Part model, mm, in its own coordinate system. A direction names the side the tool comes from. Round coordinates to 2 decimals unless told otherwise and drop trailing zeros. Write each loop counter-clockwise with the first axis right and the second up, starting at its lowest first coordinate (ties: lowest second). Pieces come first, ordered by that corner, then holes. Notation, with made-up numbers: (10.25, 63) -> (59.25, 63) arc R20 cw to (59.25, 92) -> close; hole circle Ø8 at (51.5, 48.25). An arc over 180 degrees is marked (long way). Return JSON: item names as keys, results as strings. Group by question number.
(1) Tool access for faces 4 (the flat face through (0, -8, 0)), 5 (the flat face through (-2, -18, 2)), 6 (the flat face through (5, -17, 0)): list every direction of +Z, -Z, +X, -X, +Y, -Y with a clear straight run to the whole face (end or side of a thin tool).
(2) Mould opens along X. For faces 1 (the flat face through (-0.1, -17.3, -5)), 2 (the cylindrical face through (-2.44, -13.07, 0.54)), 3 (the flat face through (-5, -17, 0)) say: +X half, -X half, draft (parallel to the pull), parting line (faces both ways), or undercut.
(3) Drill centre lines: L1, parallel to Y at x = 0.5, z = 37.5; L2, parallel to X at y = -13, z = 0; L3, parallel to X at y = -10.25, z = 0. Where is each one in solid material? Low to high. Write a range as from..to.
(4) Saw through at B-B (x = 0). List the corners of the cut face in (y, z).
(5) Saw through at C-C (z = 0). List the corners of the cut face in (x, y), plus the area to 3 significant figures.
(6) Saw through at A-A (y = -15). List the corners of the cut face in (x, z).
(7) Drop flat-ended pins along their axis: pin 1 Ø2 at (x, z) = (-5, -26) entering from -Y; pin 2 Ø2 at (x, z) = (8.5, -25) entering from +Y; pin 3 Ø1.5 at (x, z) = (0, 0.5) entering from -Y. Give the stop position or say it passes through.
(8) Saw through at D-D (y = 14). List the corners of the cut face in (x, z).
from build123d import *

# Parameters (mm, degrees)
SKETCH1_R           = 17
BOSS_EXTRUDE1_DEPTH = 40
SKETCH2_W           = 10
SKETCH2_H           = 2
BOSS_EXTRUDE2_DEPTH = 5
SKETCH3_R           = 2.5
CUT_EXTRUDE1_DEPTH  = 10


with BuildPart() as part:
    # Sketch1 → Boss-Extrude1 (new, symmetric)
    with BuildSketch(Plane.XY):
        Circle(SKETCH1_R)
    extrude(amount=BOSS_EXTRUDE1_DEPTH, both=True)

    # Sketch2 → Boss-Extrude2 (add, symmetric)
    with BuildSketch(Plane.XY):
        with Locations((0, -17)):
            Rectangle(SKETCH2_W, SKETCH2_H)
    extrude(amount=BOSS_EXTRUDE2_DEPTH, both=True)

    # Sketch3 → Cut-Extrude1 (cut)
    with BuildSketch(Plane.XZ.offset(18)):
        with Locations(Location((0, 0, 0), (0, 0, 270))):
            Circle(SKETCH3_R)
    extrude(amount=-CUT_EXTRUDE1_DEPTH, mode=Mode.SUBTRACT)


solid = part.part
Computed values:
{
 "1": {"face 4": "-Y", "face 5": "+Z, -Z, +X, -X, -Y", "face 6": "+Z, -Z, +X, -Y"},
 "2": {"face 1": "draft", "face 2": "undercut", "face 3": "-X half"},
 "3": {"L1": "-16.99..16.99", "L2": "-10.95..-2.5, 2.5..10.95", "L3": "-13.56..-2.5, 2.5..13.56"},
 "4": {"outline": "(-18, -5) -> (-17, -5) -> (-17, -40) -> (17, -40) -> (17, 40) -> (-17, 40) -> (-17, 5) -> (-18, 5) -> (-18, 2.5) -> (-8, 2.5) -> (-8, -2.5) -> (-18, -2.5) -> close"},
 "5": {"outline": "(-5, -18) -> (-2.5, -18) -> (-2.5, -8) -> (2.5, -8) -> (2.5, -18) -> (5, -18) -> (5, -16.25) arc R17 ccw (long way) to (-5, -16.25) -> close", "area": "870 mm2"},
 "6": {"outline": "(-8, -40) -> (8, -40) -> (8, 40) -> (-8, 40) -> close; hole circle Ø5 at (0, 0)"},
 "7": {"pin 1": "y = -16.52", "pin 2": "y = 15.26", "pin 3": "y = -8"},
 "8": {"outline": "(-9.64, -40) -> (9.64, -40) -> (9.64, 40) -> (-9.64, 40) -> close"}
}
